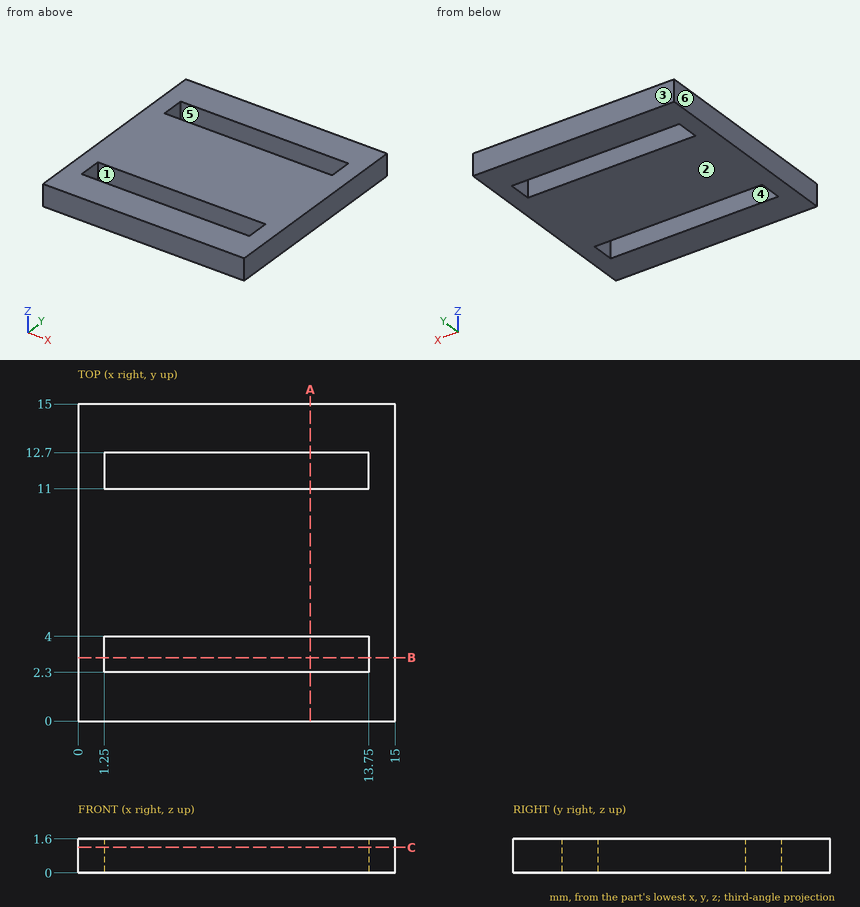
Here's the drawing with two shaded views (mm, measured from the low corner). I have some questions. A direction names the side the tool comes from. Coordinates: 2 decimals unless noted, no trailing zeros. Loops run counter-clockwise (first coordinate to the right, second up) from the corner with the lowest first, then second, coordinate; pieces in that order, holes last. Notation, with made-up numbers: (-2, -28) -> (45, -28) arc R21 cw to (45, 4) -> close; hole circle Ø1 at (42, 22.25). An arc over 180 degrees is marked (long way). Use one line per item in the form item = value. Start each with the question number.
(1) If we section it at A-A (x = 11): Please give me the cut outline in (y, z), then the cut area to 3 significant figures.
(2) If we section it at C-C (z = 1.2): Please give me the cut outline in (x, y).
(3) If we section it at B-B (y = 3): Please give me the cut outline in (x, z), then the cut area to 3 significant figures.
(4) On a 3-axis mill with a long thin cutter (end or side, diameter ignored), from which of +Z, -Z, +X, -X, +Y, -Y can I reach the whole of each face in a straight line? I mean the marked faces 1 and 2. Say none if no direction works.
(5) We'd pull the mould along X, two halves only. Please class the marked faces 3, 4, 5 and 6: pulls with the +X half, pulls with the -X half, needs draft (parallel to the pull), parting line crosses it, or undercut.
(6) Please list where these lines run through material, in increasing order: line 1 along Y through (x, z) = (2.75, 1.2); line 2 along X through (y, z) = (3.5, 0.1).
Verdict:
q1.outline = (0, 0) -> (2.3, 0) -> (2.3, 1.6) -> (0, 1.6) -> close; (4, 0) -> (11, 0) -> (11, 1.6) -> (4, 1.6) -> close; (12.7, 0) -> (15, 0) -> (15, 1.6) -> (12.7, 1.6) -> close
q1.area = 18.6 mm²
q2.outline = (0, 0) -> (15, 0) -> (15, 15) -> (0, 15) -> close; hole (1.25, 2.3) -> (13.75, 2.3) -> (13.75, 4) -> (1.25, 4) -> close; hole (1.25, 11) -> (13.75, 11) -> (13.75, 12.7) -> (1.25, 12.7) -> close
q3.outline = (0, 0) -> (1.25, 0) -> (1.25, 1.6) -> (0, 1.6) -> close; (13.75, 0) -> (15, 0) -> (15, 1.6) -> (13.75, 1.6) -> close
q3.area = 4.00 mm²
q4.face_1 = +Z, -Z
q4.face_2 = -Z, +X, -X, +Y, -Y
q5.face_3 = needs draft
q5.face_4 = undercut
q5.face_5 = undercut
q5.face_6 = pulls with the -X half
q6.line_1 = 0 to 2.3, 4 to 11, 12.7 to 15
q6.line_2 = 0 to 1.25, 13.75 to 15
